Verification items for this drawing (mm, ordinates from the low corner). A direction names the side the tool comes from. Give positions to 0.01 mm unless a question says otherwise; leave off trailing zeros. Loops run counter-clockwise (first coordinate to the right, second up) from the corner with the lowest first, then second, coordinate; pieces in that order, holes last. Notation, with made-up numbers: M 22.5,-21.75 L 69.5,-21.75 A17 ccw 69.5,2.25 Z; hole C 67,30 d6. An arc over 180 degrees is marked long. Answer in a Markdown table with one row per item.
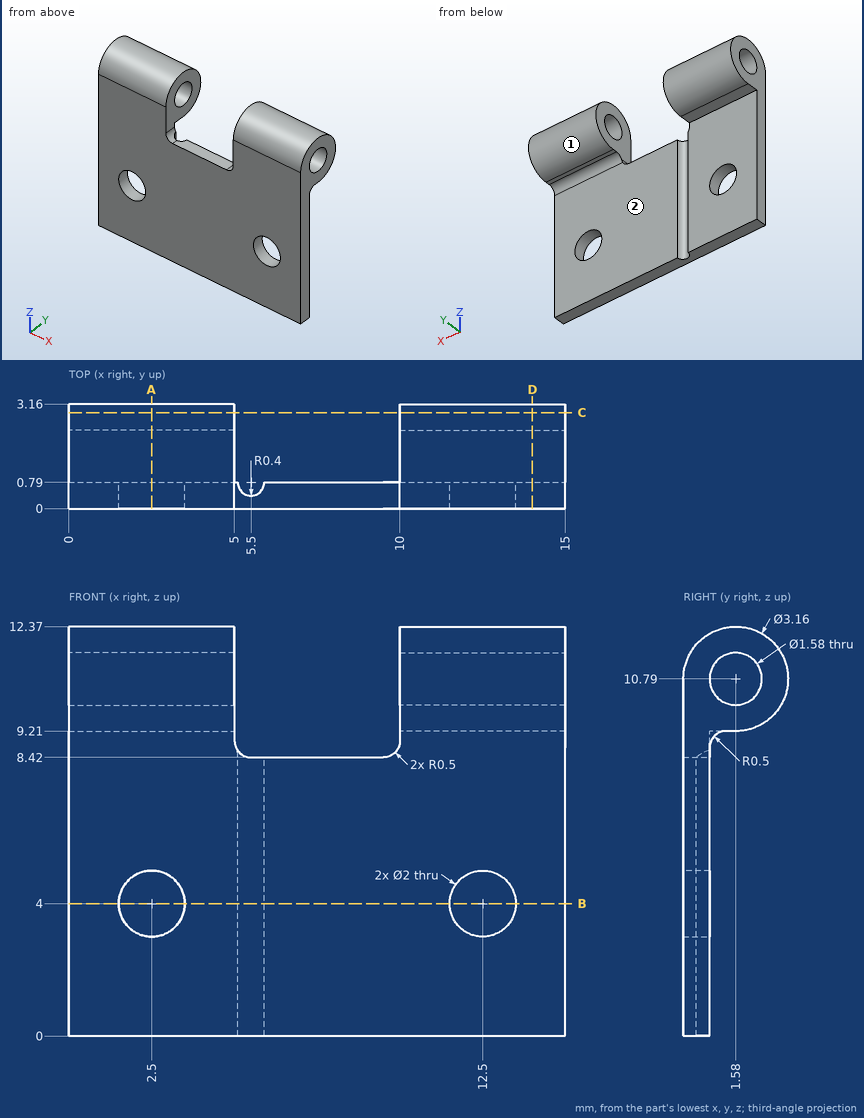
Item 1: Sectioned sample at C-C (y = 2.9). Record the cut outline in (x, z).
Reported:
| item | result |
|---|---|
| outline | M 0,9.92 L 5,9.92 L 5,11.66 L 0,11.66 Z; M 10,9.92 L 15,9.92 L 15,11.66 L 10,11.66 Z |
Item 2: Go/stop test with flat-tipped pins: pin 1 (1.5 mm diameter, centred on x = 3.5, z = 3.5, fed in from +Y); pin 2 (0.9 mm diameter, centred on x = 7, y = 0.5, fed in from +Z). Record where each tip stops, or that it passes through.
Reported:
| item | result |
|---|---|
| pin 1 | stops at y = 0.79 |
| pin 2 | stops at z = 8.42 |
Item 3: Sectioned sample at B-B (z = 4). Record the cut outline in (x, y).
Reported:
| item | result |
|---|---|
| outline | M 0,0 L 1.5,0 L 1.5,0.79 L 0,0.79 Z; M 3.5,0 L 11.5,0 L 11.5,0.79 L 5.9,0.79 A0.4 cw 5.1,0.79 L 3.5,0.79 Z; M 13.5,0 L 15,0 L 15,0.79 L 13.5,0.79 Z |
Item 4: Sectioned sample at A-A (x = 2.5). Record the cut outline in (y, z), and give its area (3 significant figures).
Reported:
| item | result |
|---|---|
| outline | M 0,0 L 0.79,0 L 0.79,3 L 0,3 Z; M 0,5 L 0.79,5 L 0.79,9.21 L 1.58,9.21 A1.58 ccw long 0,10.79 Z; hole C 1.58,10.79 d1.58 |
| area | 12.1 mm^2 |
Item 5: Scan lines: L1, parallel to X at y = 0.3, z = 4; L2, parallel to X at y = 0.6, z = 4; L3, parallel to X at y = 1.05, z = 12. Record each from-to range of solid material in increasing order. Write a range as [from, to].
Reported:
| item | result |
|---|---|
| L1 | x = [0, 1.5], [3.5, 11.5], [13.5, 15] |
| L2 | x = [0, 1.5], [3.5, 5.15], [5.85, 11.5], [13.5, 15] |
| L3 | x = [0, 5], [10, 15] |
Item 6: Sectioned sample at D-D (x = 14). Record the cut outline in (y, z), and give its area (3 significant figures).
Reported:
| item | result |
|---|---|
| outline | M 0,0 L 0.79,0 L 0.79,8.71 A0.5 cw 1.29,9.21 L 1.58,9.21 A1.58 ccw long 0,10.79 Z; hole C 1.58,10.79 d1.58 |
| area | 13.7 mm^2 |
Item 7: Tool access check on the marked faces 1 and 2. Record the directions out of +Z, -Z, +X, -X, +Y, -Y that give a thin tool (end or side, any length) a straight path to the whole face; none if there is none.
Reported:
| item | result |
|---|---|
| face 1 | +X, -X |
| face 2 | -Z, +X, -X, +Y |
